The figure shows three views and two pictorial views of one solid part (mm, origin at its lowest corner). Answer the questions. A direction names the side the tool comes from. Round coordinates to 2 decimals unless told otherwise and drop trailing zeros. Write each loop counter-clockwise with the first axis right and the second up, starting at its lowest first coordinate (ties: lowest second). Pieces come first, ordered by that corner, then holes. Notation, with made-up numbers: (49.25, 60.5) - (59.25, 60.5) arc R21 ccw to (59.25, 78.5) - close; hole circle Ø10 at (24.25, -10). An arc over 180 degrees is marked (long way). Answer as CSV lines item,"result". Start each with the question number.
Item 1: A cutting plane is placed at B-B on y = 12. Determine the outline of the cut face in (x, z).
Item 2: Straight lines are drawn through the part: line 1 along Z through (x, y) = (9.5, 9.5); line 2 along X through (y, z) = (8.5, 28); line 3 along Y through (x, z) = (13, 18.5). For each, find the intervals that lie inside material, in ascending order. Write a range as [from, to].
Item 3: Which of the six approach directions +Z, -Z, +X, -X, +Y, -Y give full straight-line access (tool end or side, diameter ignored) to the marked faces 1, 2, 3 and 4?
Item 4: A cutting plane is placed at C-C on z = 43.5. Determine the outline of the cut face in (x, y).
Item 5: A cutting plane is placed at A-A on x = 21. Determine the outline of the cut face in (y, z).
Item 6: A cutting plane is placed at D-D on x = 6.5. Determine the outline of the cut face in (y, z), and give its area (4 significant figures).
Item 7: Flat-ended cylindrical pins translate along their axes: pin 1 (2 mm diameter, centred on x = 11.5, y = 31.5, fed in from +Z); pin 2 (1 mm diameter, centred on x = 27, y = 33.5, fed in from +Z); pin 3 (4 mm diameter, centred on y = 27, z = 39, fed in from -X). Find the tip coordinate at first contact, or state that the pin passes through.
Item 8: For a pull along X with two mould halves and no side action, classify the marked faces 5, 6, 7 and 8 as pulls with the +X half, pulls with the -X half, needs draft (parallel to the pull), parting line crosses it, or undercut.
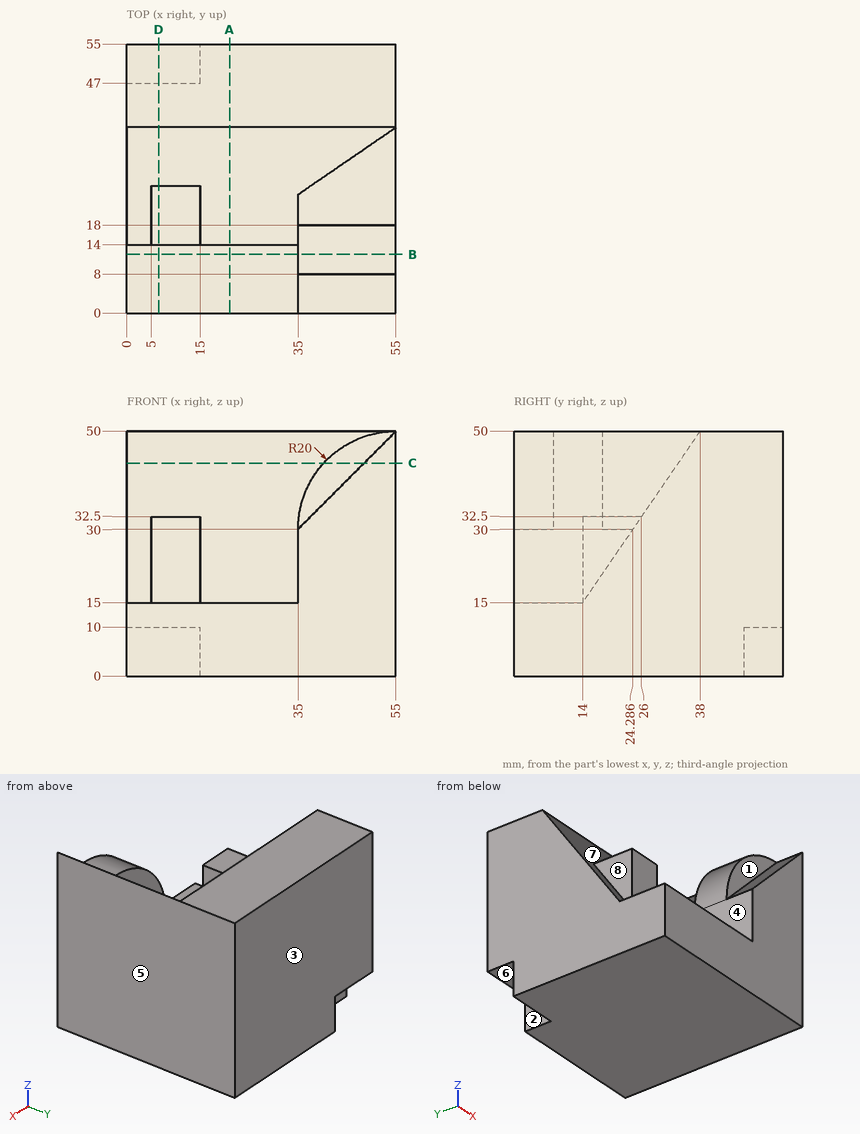
Geometry says:
1,outline,"(0, 0) - (55, 0) - (55, 50) arc R20 ccw to (35, 30) - (35, 15) - (0, 15) - close"
2,line 1,"z = [0, 15]"
2,line 2,"x = [35, 55]"
2,line 3,"y = [14, 55]"
3,face 1,"+Z, -X, -Y"
3,face 2,"-Z, -X, +Y"
3,face 3,"+Z, -Z, +X, -X, +Y"
3,face 4,"+Z, -Y"
4,outline,"(0, 33.54) - (48.5, 33.54) - (48.5, 18) - (40.24, 18) - (40.24, 8) - (48.5, 8) - (48.5, 0) - (55, 0) - (55, 55) - (0, 55) - close"
5,outline,"(0, 0) - (55, 0) - (55, 50) - (38, 50) - (14, 15) - (0, 15) - close"
6,outline,"(0, 0) - (47, 0) - (47, 10) - (55, 10) - (55, 50) - (38, 50) - (26, 32.5) - (14, 32.5) - (14, 15) - (0, 15) - close"
6,area,"1,865 mm^2"
7,pin 1,"stops at z = 41.98"
7,pin 2,"stops at z = 44.17"
7,pin 3,"stops at x = 42"
8,face 5,"pulls with the +X half"
8,face 6,"needs draft"
8,face 7,"undercut"
8,face 8,"pulls with the -X half"
